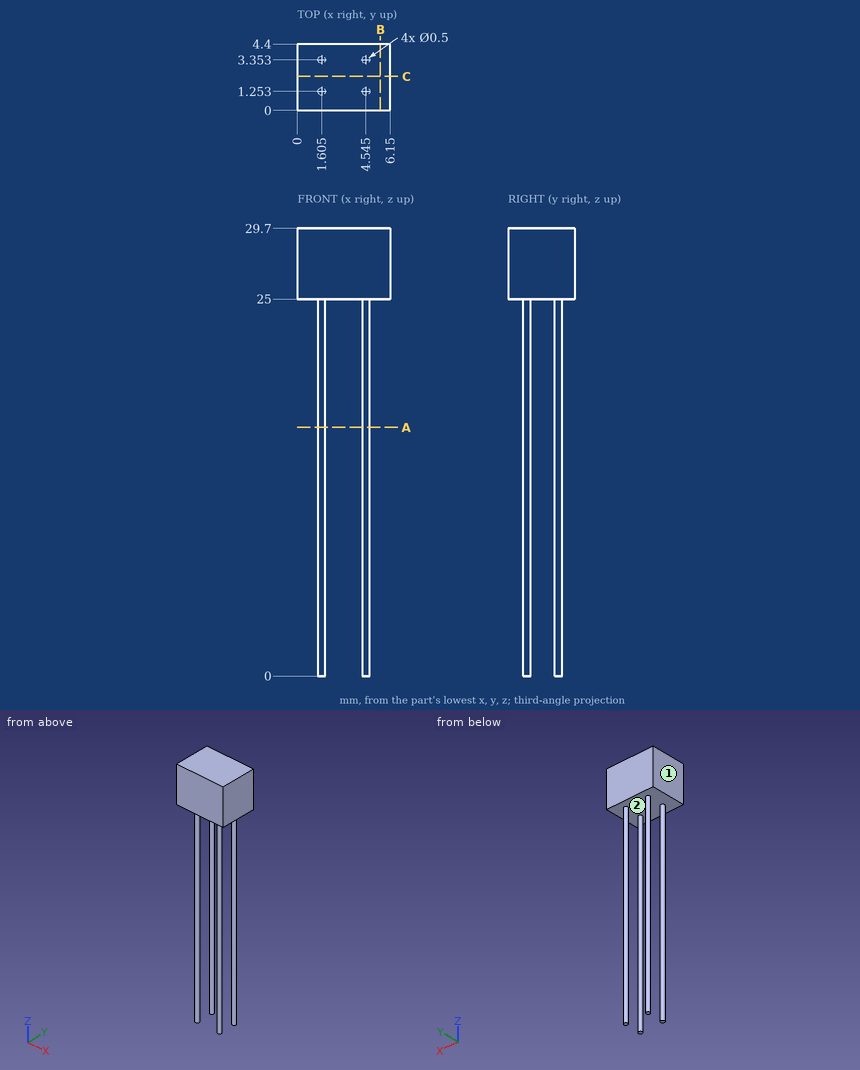
Can you work these out from the drawing? Everything is in mm from the part's minimum corner. A direction names the side the tool comes from. Coordinates: 2 decimals unless noted, no trailing zeros. Loops run counter-clockwise (first coordinate to the right, second up) from the corner with the lowest first, then second, coordinate; pieces in that order, holes last. Notation, with made-up numbers: (-12, 23.25) -> (18, 23.25) arc R22 cw to (18, 31.25) -> close; hole circle Ø9 at (62, 80). An arc over 180 degrees is marked (long way). Return JSON: item names as keys, results as strings.
1) If we section it at C-C, the plane y = 2.25: Write out the boundary of the cut face in (x, z).
Results below:
{"outline": "(0, 25) -> (6.15, 25) -> (6.15, 29.7) -> (0, 29.7) -> close"}
2) For the marked faces 1 and 2, which set-ups out of +Z, -Z, +X, -X, +Y, -Y let a thin tool reach every point of the face, with its end or its side?
Results below:
{"face 1": "+Z, -Z, -X, +Y, -Y", "face 2": "-Z"}
3) If we section it at A-A, the plane z = 16.5: Write out the boundary of the cut face in (x, y) (3 decimals).
Results below:
{"outline": "circle Ø0.5 at (1.605, 1.253); circle Ø0.5 at (1.605, 3.353); circle Ø0.5 at (4.545, 1.253); circle Ø0.5 at (4.545, 3.353)"}
4) If we section it at B-B, the plane x = 5.5: Write out the boundary of the cut face in (y, z), then the cut area to 3 significant figures.
Results below:
{"outline": "(0, 25) -> (4.4, 25) -> (4.4, 29.7) -> (0, 29.7) -> close", "area": "20.7 mm²"}
5) I need wall thicknesses on line 1 (Z direction, x = 3, y = 2.3); line 2 (X direction, y = 1.25, z = 2.75); line 3 (Y direction, x = 1.75, z = 9.75). Which ranges of each line are inside material? Lowest first, please. Write a range as from..to.
Results below:
{"line 1": "25..29.7", "line 2": "1.36..1.85, 4.3..4.79", "line 3": "1.05..1.46, 3.15..3.56"}
